Geometry check sheet. Reference: the model listing, model coordinates, mm. Face numbers are marked on the shaded views. Round coordinates to 2 decimals unless told otherwise and drop trailing zeros. Loops run counter-clockwise (first coordinate to the right, second up) from the corner with the lowest first, then second, coordinate; pieces in that order, holes last. Notation, with made-up numbers: (48, 20.25) - (91, 20.25) arc R32 ccw to (91, 57.25) - close; hole circle Ø2 at (5, 65). An arc over 180 degrees is marked (long way). Answer as CSV lines item,"result". Start each with the question number.
1) Thickness scan on line 1 along X through (y, z) = (31.5, -58); line 2 along X through (y, z) = (218.5, 237.5); line 3 along Z through (x, y) = (-88.5, 61.5). Record the ranges inside material, lowest first.
2) Cross-section at A-A on z = 16.5. Record the boundary of the cut face in (x, y), and give its area (3 significant figures).
3) Depth check by flat-ended pin: P1, Ø3, axis at y = 100.5, z = 194, coming from the +X side; P2, Ø8.5, axis at x = -62, y = 76, coming from the -Z side; P3, Ø4, axis at x = -178.5, y = -44.5, coming from the +Z side. Enter the tip coordinate at first touch or a pass-through.
4) Cross-section at B-B on z = 231. Record the boundary of the cut face in (x, y).
5) Cross-section at C-C on y = 30.5. Record the boundary of the cut face in (x, z), and give its area (3 significant figures).
6) Draft check along X on the marked faces 1, 2 and 3. Enter one of: released by +X, released by -X, zero draft, split by the parting line, or undercut.
7) Cross-section at D-D on x = -111. Record the boundary of the cut face in (y, z), and give its area (3 significant figures).
from build123d import *

# Parameters (mm, degrees)
BOSS_EXTRUDE1_DEPTH  = 90
CUT_EXTRUDE1_DEPTH   = 15
SKETCH4_W            = 3
SKETCH4_H            = 90
BOSS_EXTRUDE3_DEPTH  = 150
SKETCH5_W            = 3
SKETCH5_H            = 90
BOSS_EXTRUDE4_DEPTH  = 150
SKETCH12_W           = 20.399999779
SKETCH12_H           = 3
BOSS_EXTRUDE5_DEPTH  = 3
SKETCH13_W           = 20.399999779
SKETCH13_H           = 3
BOSS_EXTRUDE6_DEPTH  = 47
SKETCH15_W           = 3
SKETCH15_H           = 150
BOSS_EXTRUDE7_DEPTH  = 3
SKETCH16_W           = 3
SKETCH16_H           = 150
BOSS_EXTRUDE8_DEPTH  = 3
SKETCH17_W           = 3
SKETCH17_H           = 350
BOSS_EXTRUDE9_DEPTH  = 293
CUT_EXTRUDE2_DEPTH   = 263
BOSS_EXTRUDE10_DEPTH = 167.2
FILLET1_R            = 40


with BuildPart() as part:
    # Sketch2 → Boss-Extrude1 (new body)
    with BuildSketch(Plane.XY):
        Polygon((-54.932805324, 53.008197058), (-54.932805324, 97.008197058), (-72.332805103, 97.008197058), (-72.332805103, 100.008197058), (-51.932805324, 100.008197058), (-51.932805324, 50.008197058), (-72.332805103, 50.008197058), (-72.332805103, 53.008197058), align=None)
    extrude(amount=-BOSS_EXTRUDE1_DEPTH)

    # Sketch3 → Cut-Extrude1 (cut)
    with BuildSketch(Plane(origin=(-51.932805324, 0, 0), x_dir=(0, 0, -1), z_dir=(1, 0, 0))):
        with BuildLine():
            Line((25.000000095, 59.008197058), (90, 59.008197058))
            Line((90, 59.008197058), (90, 91.008197058))
            Line((90, 91.008197058), (25.000000095, 91.008197058))
            ThreePointArc((25.000000095, 91.008197058), (9.000000095, 75.008197058), (25.000000095, 59.008197058))
        make_face()
    extrude(amount=-CUT_EXTRUDE1_DEPTH, mode=Mode.SUBTRACT)

    # Sketch4 → Boss-Extrude3 (add)
    with BuildSketch(Plane.XZ.offset(-50.008197058)):
        with Locations((-70.832805103, -45)):
            Rectangle(SKETCH4_W, SKETCH4_H)
    extrude(amount=BOSS_EXTRUDE3_DEPTH)

    # Sketch5 → Boss-Extrude4 (add)
    with BuildSketch(Plane(origin=(0, 100.008197058, 0), x_dir=(1, 0, 0), z_dir=(0, 1, 0))):
        with Locations((-70.832805103, 45)):
            Rectangle(SKETCH5_W, SKETCH5_H)
    extrude(amount=BOSS_EXTRUDE4_DEPTH)

    # Sketch12 → Boss-Extrude5 (add)
    with BuildSketch(Plane.XY):
        with Locations((-62.132805213, 98.508197058)):
            Rectangle(SKETCH12_W, SKETCH12_H)
    extrude(amount=BOSS_EXTRUDE5_DEPTH)

    # Sketch13 → Boss-Extrude6 (add)
    with BuildSketch(Plane.XZ.offset(-97.008197058)):
        with Locations((-62.132805213, 1.5)):
            Rectangle(SKETCH13_W, SKETCH13_H)
    extrude(amount=BOSS_EXTRUDE6_DEPTH)

    # Sketch15 → Boss-Extrude7 (add)
    with BuildSketch(Plane.XY):
        with Locations((-70.832805103, -24.991802942)):
            Rectangle(SKETCH15_W, SKETCH15_H)
    extrude(amount=BOSS_EXTRUDE7_DEPTH)

    # Sketch16 → Boss-Extrude8 (add)
    with BuildSketch(Plane.XY):
        with Locations((-70.832805103, 175.008197058)):
            Rectangle(SKETCH16_W, SKETCH16_H)
    extrude(amount=BOSS_EXTRUDE8_DEPTH)

    # Sketch17 → Boss-Extrude9 (add)
    with BuildSketch(Plane.XY.offset(3)):
        with Locations((-70.832805103, 75.008197058)):
            Rectangle(SKETCH17_W, SKETCH17_H)
    extrude(amount=BOSS_EXTRUDE9_DEPTH)

    # Sketch18 → Cut-Extrude2 (cut)
    with BuildSketch(Plane(origin=(-69.332805103, 0, 0), x_dir=(0, 0, -1), z_dir=(1, 0, 0))):
        with BuildLine():
            Line((-218.669858525, -99.991802942), (-296, -99.991802942))
            Line((-296, -99.991802942), (-296, 250.008197058))
            Line((-296, 250.008197058), (-218.669858525, 250.008197058))
            ThreePointArc((-218.669858525, 250.008197058), (-274.999999905, 75.008197058), (-218.669858525, -99.991802942))
        make_face()
    extrude(amount=-CUT_EXTRUDE2_DEPTH, mode=Mode.SUBTRACT)


with BuildPart() as body_2:
    # Mirror3: mirrored copy
    add(part.part.mirror(Plane.ZY.offset(155.932805134)))


with BuildPart() as part_1:
    add(part.part)

    add(body_2.part)  # Boss-Extrude10 merges body 2
    # Sketch20 → Boss-Extrude10 (add)
    with BuildSketch(Plane.ZY.offset(72.332805103)):
        with BuildLine():
            Line((214.966664257, 250.008197058), (218.669858525, 250.008197058))
            ThreePointArc((218.669858525, 250.008197058), (274.999999905, 75.008197058), (218.669858525, -99.991802942))
            Line((218.669858525, -99.991802942), (214.966664257, -99.991802942))
            ThreePointArc((214.966664257, -99.991802942), (271.999999905, 75.008197058), (214.966664257, 250.008197058))
        make_face()
    extrude(amount=BOSS_EXTRUDE10_DEPTH)

    # Fillet1
    fillet1_edges = [part_1.edges().sort_by_distance(p)[0] for p in [
        (-241.032805165, 250.008197058, -90),
        (-241.032805165, -99.991802942, -90),
        (-70.832805103, -99.991802942, -90),
        (-70.832805103, 250.008197058, -90),
    ]]
    fillet(fillet1_edges, radius=FILLET1_R)


solid = part_1.part
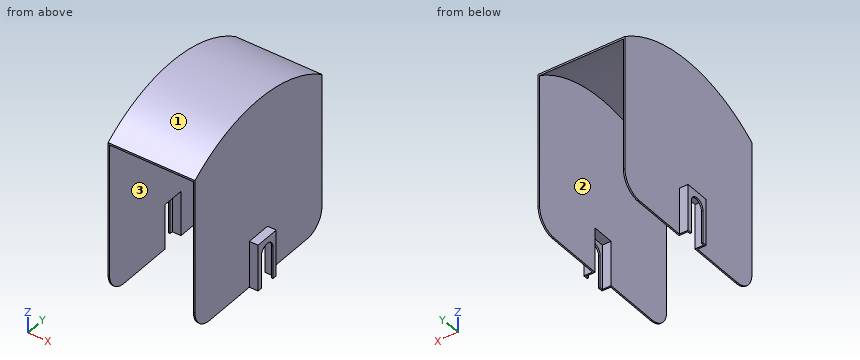
Answer block:
1,line 1,"x = -242.53 to -239.53, -72.33 to -69.33"
1,line 2,"x = -242.53 to -69.33"
1,line 3,"z = 271.69 to 274.7"
2,outline,"(-242.53, -99.99) - (-239.53, -99.99) - (-239.53, 250.01) - (-242.53, 250.01) - close; (-72.33, -99.99) - (-69.33, -99.99) - (-69.33, 250.01) - (-72.33, 250.01) - close"
2,area,"2,100 mm^2"
3,P1,"stops at x = -69.33"
3,P2,"stops at z = 0"
3,P3,"stops at z = 251.03"
4,outline,"(-242.53, -81.4) - (-69.33, -81.4) - (-69.33, 231.42) - (-242.53, 231.42) - close; hole (-239.53, -75.57) - (-72.33, -75.57) - (-72.33, 225.58) - (-239.53, 225.58) - close"
5,outline,"(-242.53, -90) - (-239.53, -90) - (-239.53, 268.65) - (-72.33, 268.65) - (-72.33, -90) - (-69.33, -90) - (-69.33, 271.68) - (-242.53, 271.68) - close"
5,area,"2,680 mm^2"
6,face 1,"zero draft"
6,face 2,"undercut"
6,face 3,"undercut"
7,outline,"(-99.99, 214.97) arc R297 cw to (250.01, 214.97) - (250.01, 218.67) arc R300 ccw to (-99.99, 218.67) - close"
7,area,"1,120 mm^2"
